Could you check a few things on this drawing? It's one solid part, dimensions in mm from its lowest x, y, z. Give positions to 0.01 mm unless a question says otherwise; leave off trailing zeros. Order: outer loops, then holes, each group sorted by start corner. A loop starts at its lowest first (then second) coordinate and runs counter-clockwise, first axis right, second up. Notation, with made-up numbers: (-5, 2) -> (34, 2) arc R27 cw to (34, 25) -> close; hole circle Ø3 at (80, 15). An arc over 180 degrees is marked (long way). Use one line per item in the form item = value. Start each with the question number.
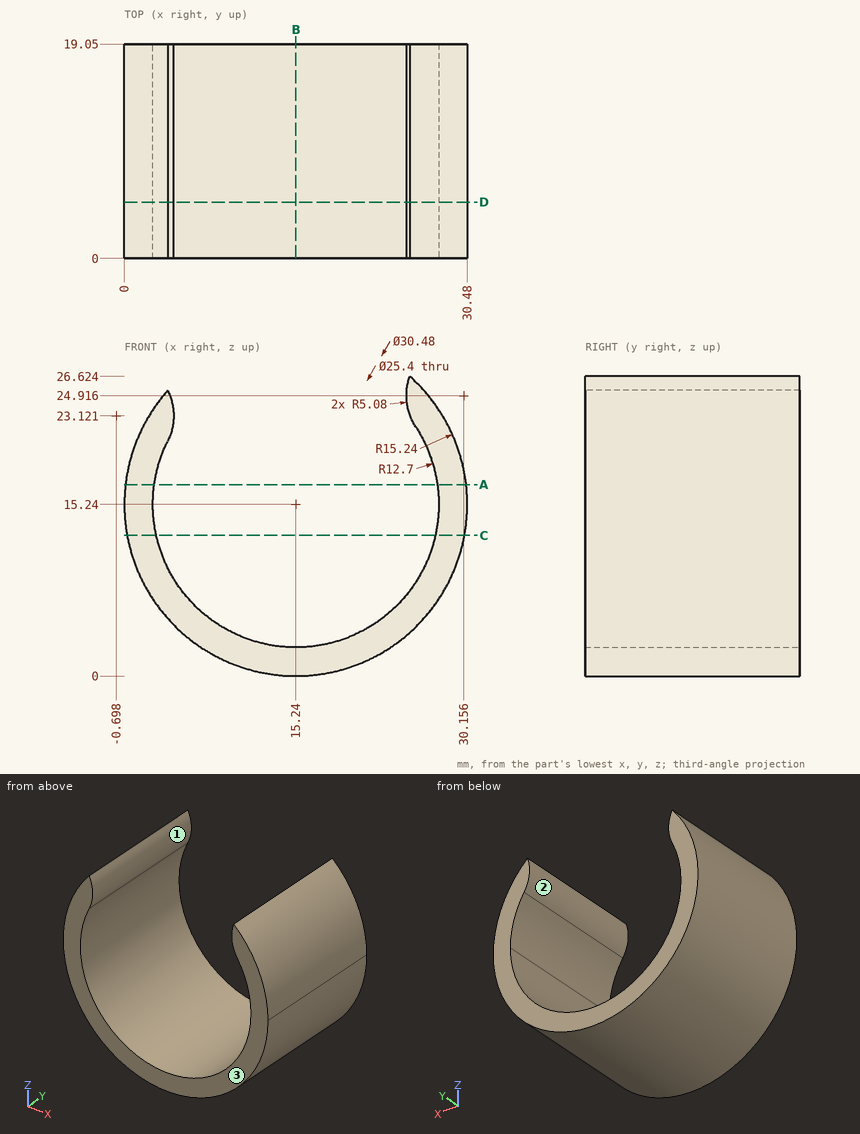
(1) Imagine slicing it at C-C (z = 12.5). Write out the boundary of the cut face in (x, y).
(2) Please list where these lines run through material, in increasing order: probe 1 along X at (y, z) = (13.75, 15.24); probe 2 along Z at (x, y) = (15.24, 14.25); probe 3 along X at (y, z) = (5.75, 5.75) (1 decimal).
(3) Imagine slicing it at A-A (z = 17). Write out the boundary of the cut face in (x, y).
(4) We'd pull the mould along X, two halves only. Please class the marked faces 1, 2 and 3: pulls with the +X half, pulls with the -X half, needs draft (parallel to the pull), parting line crosses it, or undercut.
(5) Imagine slicing it at D-D (y = 5). Write out the boundary of the cut face in (x, z) (1 decimal).
(6) Imagine slicing it at B-B (x = 15.24). Write out the boundary of the cut face in (y, z), plus the area to 3 significant figures.
(7) I'm going to push flat-ended pins straight in: pin 1 Ø8 at (x, y) = (6.5, 5) entering from +Z; pin 2 Ø5 at (y, z) = (7.5, 11) entering from +X; pin 3 Ø1.5 at (y, z) = (10, 6.5) entering from +X. Where does each tip first touch, or does it pass through?
Calculated:
q1.outline = (0.25, 0) -> (2.84, 0) -> (2.84, 19.05) -> (0.25, 19.05) -> close; (27.64, 0) -> (30.23, 0) -> (30.23, 19.05) -> (27.64, 19.05) -> close
q2.probe_1 = 0 to 2.54, 27.94 to 30.48
q2.probe_2 = 0 to 2.54
q2.probe_3 = 3.3 to 6.8, 23.7 to 27.2
q3.outline = (0.1, 0) -> (2.66, 0) -> (2.66, 19.05) -> (0.1, 19.05) -> close; (27.82, 0) -> (30.38, 0) -> (30.38, 19.05) -> (27.82, 19.05) -> close
q4.face_1 = undercut
q4.face_2 = undercut
q4.face_3 = needs draft
q5.outline = (3.9, 20.9) arc R5.1 ccw to (3.9, 25.4) arc R15.2 ccw (long way) to (25.4, 26.6) arc R5.1 ccw to (25.9, 22.2) arc R12.7 cw (long way) to start
q6.outline = (0, 0) -> (19.05, 0) -> (19.05, 2.54) -> (0, 2.54) -> close
q6.area = 48.4 mm2
q7.pin_1 = 25.37
q7.pin_2 = 30.38
q7.pin_3 = 28.22
